Drawing for the job (mm, zero at the part's lowest x, y, z). Give positions to 0.01 mm unless a question says otherwise; leave off trailing zeros. Order: outer loops, then holes, each group sorted by start corner. A loop starts at its lowest first (then second) coordinate and runs counter-clockwise, first axis right, second up. Notation, with made-up numbers: (-7.5, 88.5) - (0.5, 88.5) arc R33 cw to (0.5, 117.5) - close; hole circle Ø10 at (-12, -22.5). An arc over 180 degrees is marked (long way). Use CSV: the item, a comma, the result in double quotes. Start each with the question number.
(1) Pull direction X, two halves, no side cores. Call the marked faces 1, 2 and 3: +X half, -X half, draft (parallel to the pull), parting line (faces both ways), or undercut.
(2) Band-saw the part on D-D, the plane y = 6. Give the cut face in (x, z), then the cut area to 3 significant figures.
(3) Drop a flat-ended pin along its axis: pin 1 Ø1.5 at (x, y) = (0.5, 3.5) entering from +Z. Give the stop position or say it passes through.
(4) Probe L1, parallel to Z at x = 1.5, y = 4.55; L2, parallel to Z at x = 1.95, y = 3; L3, parallel to X at y = 5, z = 1.6. List the from-to ranges inside material, lowest first.
(5) Band-saw the part on B-B, the plane z = 1.2. Give the cut face in (x, y).
(6) Band-saw the part on C-C, the plane y = 1.5. Give the cut face in (x, z).
(7) Band-saw the part on A-A, the plane x = 1.5. Give the cut face in (y, z).
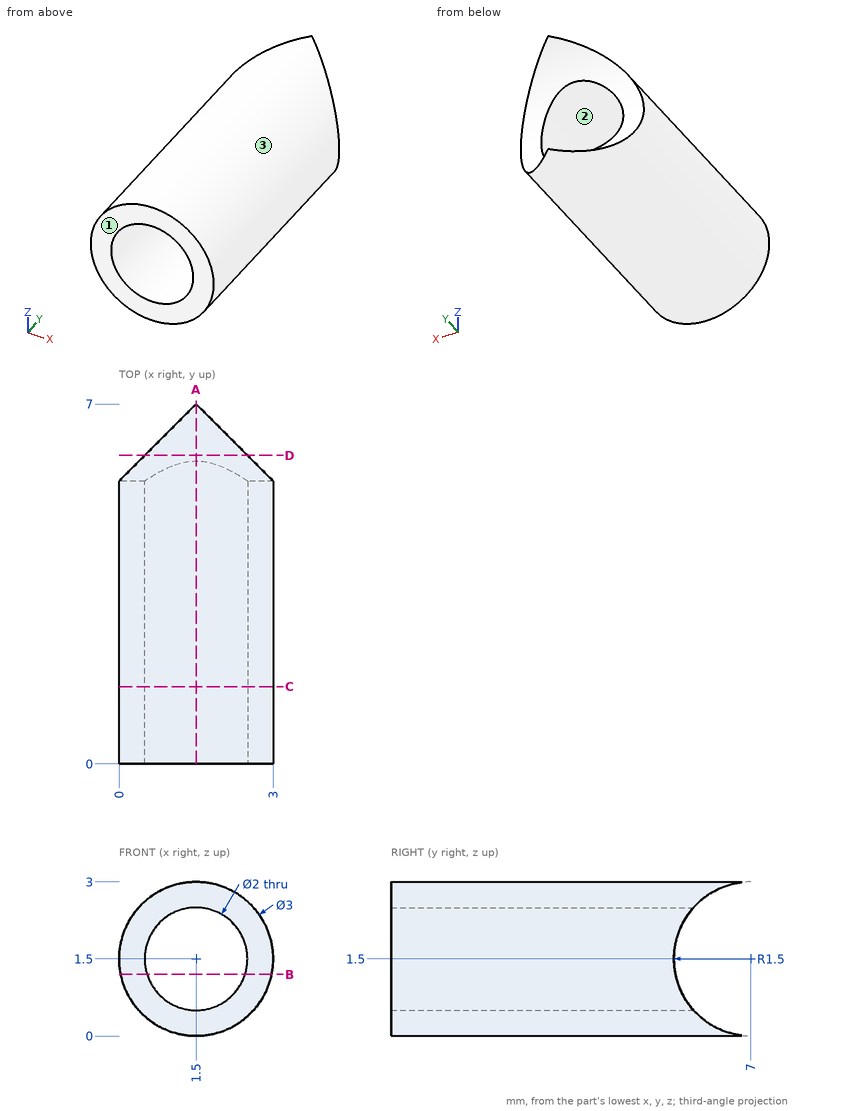
Answer block:
1,face 1,"draft"
1,face 2,"undercut"
1,face 3,"parting line"
2,outline,"(0.5, 0.38) arc R1.5 ccw to (2.5, 0.38) - close; (0.5, 2.62) - (2.5, 2.62) arc R1.5 ccw to start"
2,area,"1.05 mm2"
3,pin 1,"stops at z = 2.98"
4,L1,"z = 0 to 0.5, 2.5 to 3"
4,L2,"z = 0.07 to 0.61, 2.39 to 2.93"
4,L3,"x = 0 to 0.51, 2.49 to 3"
5,outline,"(0.03, 0) - (0.55, 0) - (0.55, 5.53) - (0.03, 5.53) - close; (2.45, 0) - (2.97, 0) - (2.97, 5.53) - (2.45, 5.53) - close"
6,outline,"circle Ø3 at (1.5, 1.5); hole circle Ø2 at (1.5, 1.5)"
7,outline,"(0, 0) - (7, 0) arc R1.5 cw to (5.88, 0.5) - (0, 0.5) - close; (0, 2.5) - (5.88, 2.5) arc R1.5 cw to (7, 3) - (0, 3) - close"
